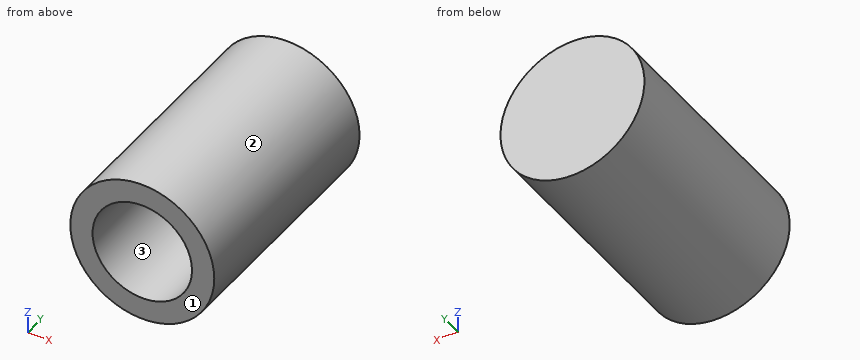
Autodesk Fusion 360 part; units mm, degrees
sketch "Esboço1" plane through (0, 0, 0) normal (0, 1, 0) x (1, 0, 0)
cylinder "Cilindro primitivo1" add diameter 5.5 height 9 placed x (1, 0, 0) y (0, 0, -1) z (0, 1, 0) at (0, 0, 0) makes body 1
cylinder "Cilindro primitivo2" cut diameter 3.8 height 3.8 placed x (1, 0, 0) y (0, 0, -1) z (0, 1, 0) at (0, 0, 0) bodies 1
copy_body "Corpo -> Componente1" bodies 1 removing the originals makes body 2 in component "Component'"
component "Component'" placed x (1, 0, 0) y (0, 1, 0) z (0, 0, 1) at (0, 0, 0)
Check sheet for the modelled part. Datum: model origin and axes. Units: mm. Face numbers are marked on the shaded views. Coordinates: 2 decimals unless noted, no trailing zeros. Order: outer loops, then holes, each group sorted by start corner. A loop starts at its lowest first (then second) coordinate and runs counter-clockwise, first axis right, second up. Notation, with made-up numbers: M 4,45.5 L 48,45.5 A24 ccw 48,70.5 Z; hole C 34,14.5 d9. An arc over 180 degrees is marked long. Write each question's results on one line, items separated by ' | '. Start each with the question number.
1. Cross-section at C-C on z = 0. Record the cut outline in (x, y).
2. Cross-section at B-B on y = 0.5. Record the cut outline in (x, z).
3. Go/stop test with flat-tipped pins: P1, Ø2, axis at x = 1.5, y = 2, coming from the -Z side; P2, Ø3, axis at x = 0, z = 0, coming from the -Y side; P3, Ø2, axis at y = 2.5, z = 2, coming from the +X side. Record where each tip stops, or that it passes through.
4. Cross-section at D-D on y = 6.5. Record the cut outline in (x, z).
5. Cross-section at A-A on x = 0. Record the cut outline in (y, z), and give its area (3 significant figures).
6. Mould release check, pull along Z, two halves, no side actions. Record for the marked faces 1, 2 and 3: +Z half, -Z half, draft (parallel to the pull), parting line (faces both ways), or undercut.
7. Material ranges on probe 1 along X at (y, z) = (1.35, 0); probe 2 along Y at (x, z) = (0.7, -0.75), recorded low to high.
Checks:
1) outline: M -2.75,0 L -1.9,0 L -1.9,3.8 L 1.9,3.8 L 1.9,0 L 2.75,0 L 2.75,9 L -2.75,9 Z
2) outline: C 0,0 d5.5; hole C 0,0 d3.8
3) P1: stops at z = -2.7 | P2: stops at y = 3.8 | P3: stops at x = 2.56
4) outline: C 0,0 d5.5
5) outline: M 0,-2.75 L 9,-2.75 L 9,2.75 L 0,2.75 L 0,1.9 L 3.8,1.9 L 3.8,-1.9 L 0,-1.9 Z | area: 35.1 mm²
6) face 1: draft | face 2: parting line | face 3: undercut
7) probe 1: x = -2.75 to -1.9, 1.9 to 2.75 | probe 2: y = 3.8 to 9
